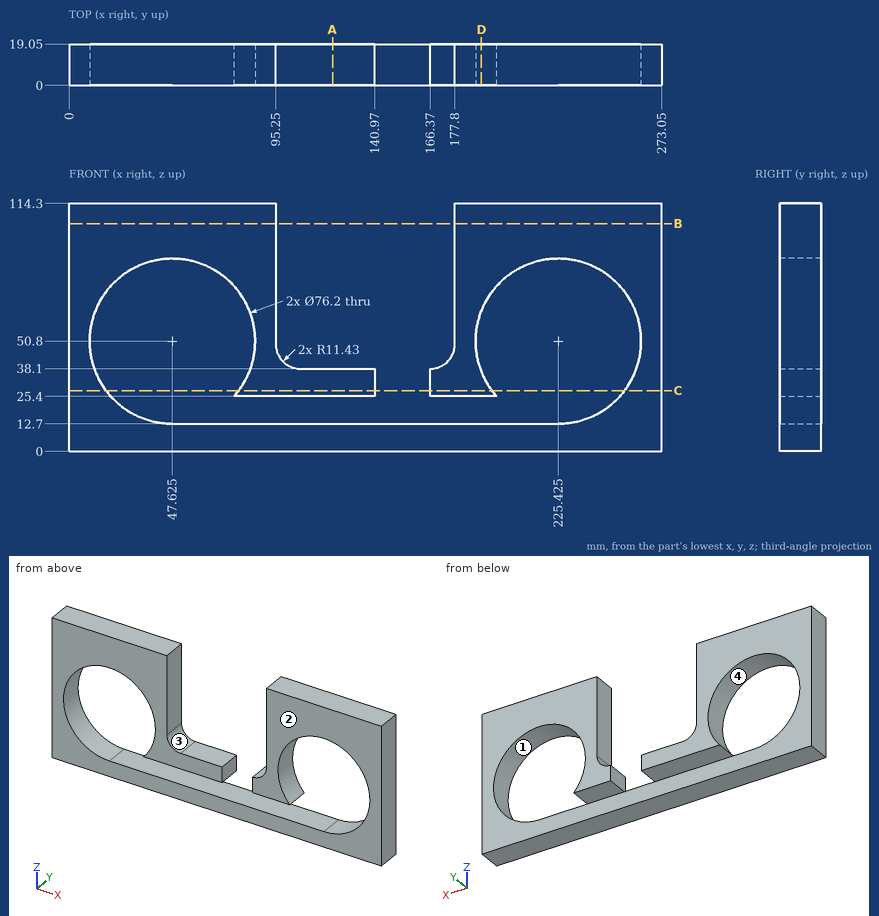
Design review of the part shown in the three views and the two pictorial views. Dimensions are in mm from the part's minimum x, y and z. Round coordinates to 2 decimals unless told otherwise and drop trailing zeros. Order: outer loops, then holes, each group sorted by start corner. A loop starts at its lowest first (then second) coordinate and runs counter-clockwise, first axis right, second up.
(1) Take a section at A-A, the plane x = 121.5. State the section outline as (y, z) points, plus the area to 3 significant figures.
Working result:
outline: (0, 0) - (19.05, 0) - (19.05, 12.7) - (0, 12.7) - close; (0, 25.4) - (19.05, 25.4) - (19.05, 38.1) - (0, 38.1) - close
area: 484 mm2
(2) Wall thickness on L1, parallel to X at y = 8, z = 50.8 (3 decimals); L2, parallel to Z at x = 111, y = 13.5; L3, parallel to X at y = 13.5, z = 67.5: over which ranges is each line inside the solid? List them lowest first.
Working result:
L1: x = 0 to 9.525, 85.725 to 95.25, 177.8 to 187.325, 263.525 to 273.05
L2: z = 0 to 12.7, 25.4 to 38.1
L3: x = 0 to 13.38, 81.87 to 95.25, 177.8 to 191.18, 259.67 to 273.05
(3) Take a section at C-C, the plane z = 28. State the section outline as (x, y) points, plus the area to 3 significant figures.
Working result:
outline: (0, 0) - (17.1, 0) - (17.1, 19.05) - (0, 19.05) - close; (78.15, 0) - (140.97, 0) - (140.97, 19.05) - (78.15, 19.05) - close; (166.37, 0) - (194.9, 0) - (194.9, 19.05) - (166.37, 19.05) - close; (255.95, 0) - (273.05, 0) - (273.05, 19.05) - (255.95, 19.05) - close
area: 2,390 mm2
(4) Take a section at D-D, the plane x = 190. State the section outline as (y, z) points.
Working result:
outline: (0, 0) - (19.05, 0) - (19.05, 12.7) - (0, 12.7) - close; (0, 25.4) - (19.05, 25.4) - (19.05, 36.78) - (0, 36.78) - close; (0, 64.82) - (19.05, 64.82) - (19.05, 114.3) - (0, 114.3) - close
(5) For P1, Ø8, axis at x = 169, y = 11, coming from the +Z side; P2, Ø5.5, axis at x = 122.5, y = 12, coming from the +Z side, all flat-tipped, find the tip position at first contact; note any pin that passes through.
Working result:
P1: stops at z = 40.22
P2: stops at z = 38.1
(6) Mouldability with a two-part tool opening along Z and no side actions: class the marked faces 1, 2, 3 and 4 as released by +Z, released by -Z, zero draft, split by the parting line, or undercut.
Working result:
face 1: undercut
face 2: zero draft
face 3: released by +Z
face 4: undercut
(7) Take a section at B-B, the plane z = 105. State the section outline as (x, y) points.
Working result:
outline: (0, 0) - (95.25, 0) - (95.25, 19.05) - (0, 19.05) - close; (177.8, 0) - (273.05, 0) - (273.05, 19.05) - (177.8, 19.05) - close
